Verification items for the finished model (mm, model axes). A direction names the side the tool comes from. Give positions to 0.01 mm unless a question says otherwise; leave off trailing zeros. Write each loop counter-clockwise with the first axis right and the second up, starting at its lowest first coordinate (ties: lowest second). Pieces come first, ordered by that corner, then holes. Notation, with made-up numbers: M 8.5,80 L 46.5,80 A17 cw 46.5,87 Z; hole C 30,-2 d4. An arc over 180 degrees is marked long. Write item = value, one per line.
from build123d import *

# Parameters (mm, degrees)
SKETCH2_W           = 107
SKETCH2_H           = 7.924066875
BOSS_EXTRUDE1_DEPTH = 48.42
FILLET1_R           = 3
SKETCH3_W           = 112.08
SKETCH3_H           = 13.004066875
BOSS_EXTRUDE2_DEPTH = 2.54
SKETCH4_W           = 112.08
SKETCH4_H           = 13.004066875
BOSS_EXTRUDE3_DEPTH = 2.54
FILLET2_R           = 3


with BuildPart() as part:
    # Sketch2 → Boss-Extrude1 (new body)
    with BuildSketch(Plane.XY):
        with Locations((53.5, 3.962033438)):
            Rectangle(SKETCH2_W, SKETCH2_H)
    extrude(amount=BOSS_EXTRUDE1_DEPTH)

    # Fillet1
    fillet1_edges = [part.edges().sort_by_distance(p)[0] for p in [
        (0, 0, 24.21),
        (0, 7.924066875, 24.21),
        (107, 7.924066875, 24.21),
        (107, 0, 24.21),
    ]]
    fillet(fillet1_edges, radius=FILLET1_R)

    # Sketch3 → Boss-Extrude2 (add)
    with BuildSketch(Plane.XY.offset(48.42)):
        with Locations((53.5, 3.962033438)):
            Rectangle(SKETCH3_W, SKETCH3_H)
    extrude(amount=BOSS_EXTRUDE2_DEPTH)

    # Sketch4 → Boss-Extrude3 (add)
    with BuildSketch(Plane(origin=(0, 0, 0), x_dir=(-1, 0, 0), z_dir=(0, 0, -1))):
        with Locations((-53.5, 3.962033438)):
            Rectangle(SKETCH4_W, SKETCH4_H)
    extrude(amount=BOSS_EXTRUDE3_DEPTH)

    # Fillet2
    fillet2_edges = [part.edges().sort_by_distance(p)[0] for p in [
        (-2.54, 10.464066875, 49.69),
        (-2.54, -2.54, 49.69),
        (109.54, -2.54, 49.69),
        (109.54, 10.464066875, 49.69),
        (109.54, 10.464066875, -1.27),
        (109.54, -2.54, -1.27),
        (-2.54, -2.54, -1.27),
        (-2.54, 10.464066875, -1.27),
    ]]
    fillet(fillet2_edges, radius=FILLET2_R)


solid = part.part
1) Material ranges on probe 1 along Z at (x, y) = (101, 9.5); probe 2 along Y at (x, z) = (49, 20); probe 3 along X at (y, z) = (4.5, 8.5), recorded low to high. Write a range as from..to.
From the geometry:
probe_1 = -2.54..0, 48.42..50.96
probe_2 = 0..7.92
probe_3 = 0..107
2) Cross-section at A-A on y = 9. Record the boundary of the cut face in (x, z), plus the area to 3 significant figures.
From the geometry:
outline = M -2.12,-2.54 L 109.12,-2.54 L 109.12,0 L -2.12,0 Z; M -2.12,48.42 L 109.12,48.42 L 109.12,50.96 L -2.12,50.96 Z
area = 565 mm^2
3) Cross-section at B-B on z = 2. Record the boundary of the cut face in (x, y).
From the geometry:
outline = M 0,3 A3 ccw 3,0 L 104,0 A3 ccw 107,3 L 107,4.92 A3 ccw 104,7.92 L 3,7.92 A3 ccw 0,4.92 Z
4) Depth check by flat-ended pin: P1, Ø0.6, axis at y = 3.5, z = 24.5, coming from the +X side; P2, Ø14.5, axis at x = 50, z = 25, coming from the +Y side; P3, Ø3, axis at y = 6.5, z = 32.5, coming from the -X side. Enter the tip coordinate at first touch or a pass-through.
From the geometry:
P1 = 107
P2 = 7.92
P3 = 0
5) Draft check along Z on faces 1 (the flat face through (53, 4, 50.96)), 2 (the flat face through (54.3, -0.3, 0)), 3 (the cylindrical face through (-1.685, 9.562, 49.708)). Enter one of: +Z half, -Z half, draft (parallel to the pull), parting line (faces both ways), or undercut.
From the geometry:
face_1 = +Z half
face_2 = undercut
face_3 = draft
6) Tool access check on faces 4 (the cylindrical face through (106.145, 7.022, 24.549)), 5 (the cylindrical face through (106.1, 0.86, 24.55)), 6 (the flat face through (53, 7.924, 24)). Record the directions out of +Z, -Z, +X, -X, +Y, -Y that give a thin tool (end or side, any length) a straight path to the whole face; none if there is none.
From the geometry:
face_4 = +X, +Y
face_5 = +X, -Y
face_6 = +X, -X, +Y
7) Cross-section at C-C on x = 94.5. Record the boundary of the cut face in (y, z).
From the geometry:
outline = M -2.54,-2.54 L 10.46,-2.54 L 10.46,0 L 7.92,0 L 7.92,48.42 L 10.46,48.42 L 10.46,50.96 L -2.54,50.96 L -2.54,48.42 L 0,48.42 L 0,0 L -2.54,0 Z
